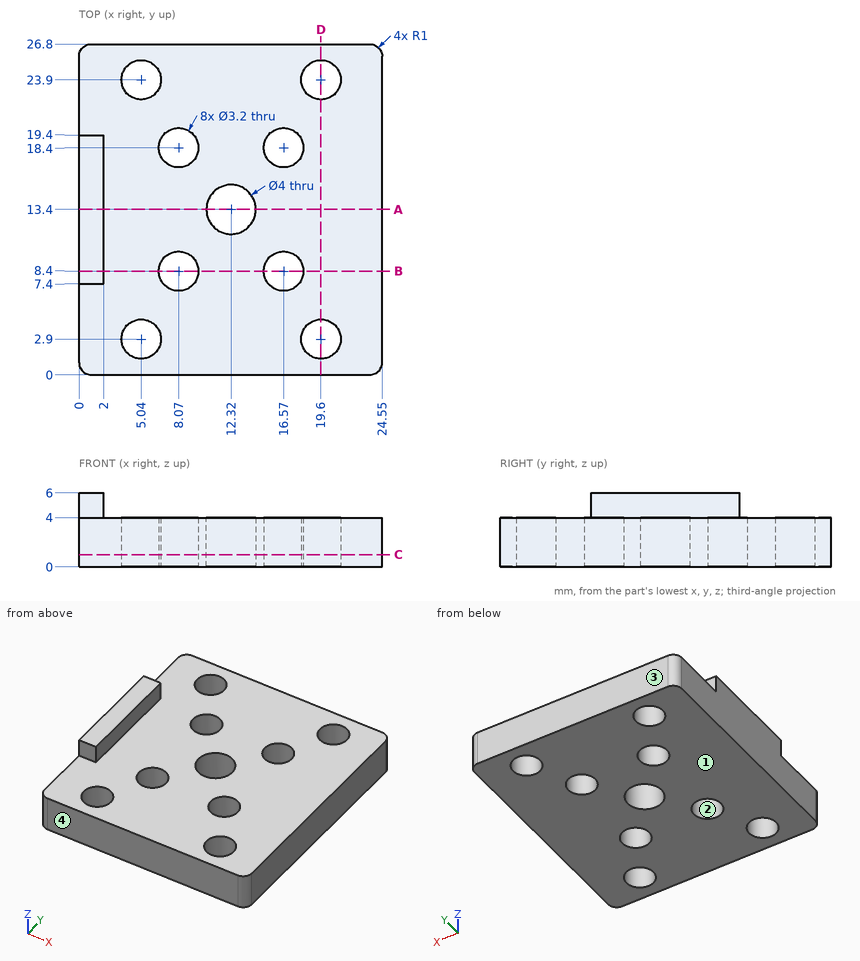
Print and shaded views of the part. All mm, measured from the part's lowest x, y and z. Coordinates: 2 decimals unless noted, no trailing zeros. Loops run counter-clockwise (first coordinate to the right, second up) from the corner with the lowest first, then second, coordinate; pieces in that order, holes last. Notation, with made-up numbers: (11, -3) -> (64, -3) arc R23 cw to (64, 24) -> close; hole circle Ø10 at (61.25, 71.25). An arc over 180 degrees is marked (long way). Use a Markdown table: item, result. Add a question column.
Item 1: Band-saw the part on A-A on y = 13.4. Write the cut outline in (x, z).
Item 2: Band-saw the part on B-B on y = 8.4. Write the cut outline in (x, z).
Item 3: Flat gauge pins, fed straight in: P1, Ø1.6, axis at x = 1, z = 5, coming from the -Y side; P2, Ø12.5, axis at x = 12.5, y = 11, coming from the +Z side; P3, Ø1, axis at x = 1, z = 5, coming from the +Y side. Where does each tip first touch, or does it go through?
Item 4: Probe probe 1 along Y at (x, z) = (16.57, 2.6); probe 2 along Y at (x, z) = (19.6, 2.95); probe 3 along Y at (x, z) = (12.32, 1.7). List the from-to ranges inside material, lowest first.
Item 5: Band-saw the part on D-D on x = 19.6. Write the cut outline in (y, z).
Item 6: Pull direction Y, two halves, no side cores. Call the marked faces 1, 2, 3 and 4: +Y half, -Y half, draft (parallel to the pull), parting line (faces both ways), or undercut.
Item 7: Band-saw the part on C-C on z = 1. Give the number of separate pieces and of enclosed holes in the cut face, plus the area to 3 significant figures.
Geometry says:
| question | item | result |
|---|---|---|
| 1 | outline | (0, 0) -> (10.32, 0) -> (10.32, 4) -> (2, 4) -> (2, 6) -> (0, 6) -> close; (14.32, 0) -> (24.55, 0) -> (24.55, 4) -> (14.32, 4) -> close |
| 2 | outline | (0, 0) -> (6.47, 0) -> (6.47, 4) -> (2, 4) -> (2, 6) -> (0, 6) -> close; (9.67, 0) -> (14.97, 0) -> (14.97, 4) -> (9.67, 4) -> close; (18.17, 0) -> (24.55, 0) -> (24.55, 4) -> (18.17, 4) -> close |
| 3 | P1 | y = 7.4 |
| 3 | P2 | z = 4 |
| 3 | P3 | y = 19.4 |
| 4 | probe 1 | 0 to 6.8, 10 to 16.8, 20 to 26.8 |
| 4 | probe 2 | 0 to 1.3, 4.5 to 22.3, 25.5 to 26.8 |
| 4 | probe 3 | 0 to 11.4, 15.4 to 26.8 |
| 5 | outline | (0, 0) -> (1.3, 0) -> (1.3, 4) -> (0, 4) -> close; (4.5, 0) -> (22.3, 0) -> (22.3, 4) -> (4.5, 4) -> close; (25.5, 0) -> (26.8, 0) -> (26.8, 4) -> (25.5, 4) -> close |
| 6 | face 1 | draft |
| 6 | face 2 | undercut |
| 6 | face 3 | +Y half |
| 6 | face 4 | -Y half |
| 7 | separate pieces | 1 |
| 7 | enclosed holes | 9 |
| 7 | area | 580 mm² |
